from build123d import *

# Parameters (mm, degrees)
SZKIC1_R                    = 49
SZKIC1_R_2                  = 34.5
DODANIE_WYCI_GNI_CIE1_DEPTH = 15
SZKIC2_R                    = 3.3
WYTNIJ_WYCI_GNI_CIE1_DEPTH  = 6
SZYK_KO_OWY1_COUNT          = 6
SZKIC3_R                    = 39
WYTNIJ_WYCI_GNI_CIE2_DEPTH  = 10


with BuildPart() as part:
    # Szkic1 → Dodanie-wyciągnięcie1 (new body)
    with BuildSketch(Plane.XY):
        Circle(SZKIC1_R)
        Circle(SZKIC1_R_2, mode=Mode.SUBTRACT)
    extrude(amount=DODANIE_WYCI_GNI_CIE1_DEPTH)

    # Szkic2 → Wytnij-wyciągnięcie1 (cut)
    with BuildSketch(Plane(origin=(0, 0, 0), x_dir=(-1, 0, 0), z_dir=(0, 0, -1))):
        with Locations((44, 0)):
            Circle(SZKIC2_R)
    wytnij_wyci_gni_cie1 = extrude(amount=-WYTNIJ_WYCI_GNI_CIE1_DEPTH, mode=Mode.SUBTRACT)

    # Szyk kołowy1: Wytnij-wyciągnięcie1 ×6 about axis
    szyk_ko_owy1_axis = Axis((0, 0, 0), (0, 0, 1))
    for i in range(1, SZYK_KO_OWY1_COUNT):
        add(wytnij_wyci_gni_cie1.rotate(szyk_ko_owy1_axis, i * 360 / SZYK_KO_OWY1_COUNT), mode=Mode.SUBTRACT)

    # Szkic3 → Wytnij-wyciągnięcie2 (cut)
    with BuildSketch(Plane.XY.offset(15)):
        Circle(SZKIC3_R)
    extrude(amount=-WYTNIJ_WYCI_GNI_CIE2_DEPTH, mode=Mode.SUBTRACT)


solid = part.part
Could you check a few things on this model? Use its own coordinates, in mm. A direction names the side the tool comes from. Round coordinates to 2 decimals unless told otherwise and drop trailing zeros. Write each loop counter-clockwise with the first axis right and the second up, starting at its lowest first coordinate (ties: lowest second). Pieces come first, ordered by that corner, then holes. Notation, with made-up numbers: (43, 58.25) - (91, 58.25) arc R22 ccw to (91, 95.25) - close; hole circle Ø2 at (-19.5, -37.5). An arc over 180 degrees is marked (long way). Use a Markdown table: item, result.
Q1. I want a section at A-A (x = 0). List the corners of the cut face in (y, z) for me, plus the area to 3 significant figures.
Output values:
| item | result |
|---|---|
| outline | (-49, 0) - (-34.5, 0) - (-34.5, 5) - (-39, 5) - (-39, 15) - (-49, 15) - close; (34.5, 0) - (49, 0) - (49, 15) - (39, 15) - (39, 5) - (34.5, 5) - close |
| area | 345 mm2 |
Q2. Please list where these lines run through material, in increasing order: L1, parallel to X at y = 27.5, z = 8; L2, parallel to X at y = 23, z = 13.25; L3, parallel to Y at x = -32, z = 12.
Output values:
| item | result |
|---|---|
| L1 | -40.56 to -27.65, 27.65 to 40.56 |
| L2 | -43.27 to -31.5, 31.5 to 43.27 |
| L3 | -37.11 to -22.29, 22.29 to 37.11 |
Q3. For pin 1 (1 mm diameter, centred on y = -18.5, z = 11, fed in from -X); pin 2 (5.5 mm diameter, centred on x = -22, y = 38.11, fed in from -Z); pin 3 (1.5 mm diameter, centred on y = -7.5, z = 8.5, fed in from -X), each with a flat end and sliding along its axis, tell me the tip position at first contact or that it passes through.
Output values:
| item | result |
|---|---|
| pin 1 | x = -45.57 |
| pin 2 | z = 6 |
| pin 3 | x = -48.53 |
Q4. I want a section at B-B (y = 17.5). List the corners of the cut face in (x, z) for me.
Output values:
| item | result |
|---|---|
| outline | (-45.77, 0) - (-29.73, 0) - (-29.73, 5) - (-34.85, 5) - (-34.85, 15) - (-45.77, 15) - close; (29.73, 0) - (45.77, 0) - (45.77, 15) - (34.85, 15) - (34.85, 5) - (29.73, 5) - close |
Q5. For faces 4 (the flat face through (-33.4, -10.2, 0)), 5 (the flat face through (-22, 38, 6)), 6 (the cylindrical face through (-5.077, 38.668, 10.07)), which set-ups out of +Z, -Z, +X, -X, +Y, -Y let a thin tool reach every point of the face, with its end or its side?
Output values:
| item | result |
|---|---|
| face 4 | -Z, +X, -X, +Y, -Y |
| face 5 | -Z |
| face 6 | +Z |
Q6. I want a section at C-C (z = 2.75). List the corners of the cut face in (x, y) for me.
Output values:
| item | result |
|---|---|
| outline | circle Ø98 at (0, 0); hole circle Ø6.6 at (-44, 0); hole circle Ø69 at (0, 0); hole circle Ø6.6 at (-22, -38.11); hole circle Ø6.6 at (-22, 38.11); hole circle Ø6.6 at (22, -38.11); hole circle Ø6.6 at (22, 38.11); hole circle Ø6.6 at (44, 0) |
Q7. I want a section at D-D (x = 22). List the corners of the cut face in (y, z) for me, plus the area to 3 significant figures.
Output values:
| item | result |
|---|---|
| outline | (-43.78, 0) - (-41.41, 0) - (-41.41, 6) - (-34.81, 6) - (-34.81, 0) - (-26.58, 0) - (-26.58, 5) - (-32.2, 5) - (-32.2, 15) - (-43.78, 15) - close; (26.58, 0) - (34.81, 0) - (34.81, 6) - (41.41, 6) - (41.41, 0) - (43.78, 0) - (43.78, 15) - (32.2, 15) - (32.2, 5) - (26.58, 5) - close |
| area | 325 mm2 |
Q8. Thinking about a two-plate mould opening in Y: for faces 1 (the flat face through (-33, -22, 15)), 2 (the cylindrical face through (40.7, -0.1, 3)), 3 (the cylindrical face through (26.34, 41.32, 7.4)), which applies, released by +Y, released by -Y, zero draft, split by the parting line, or undercut?
Output values:
| item | result |
|---|---|
| face 1 | zero draft |
| face 2 | undercut |
| face 3 | split by the parting line |
